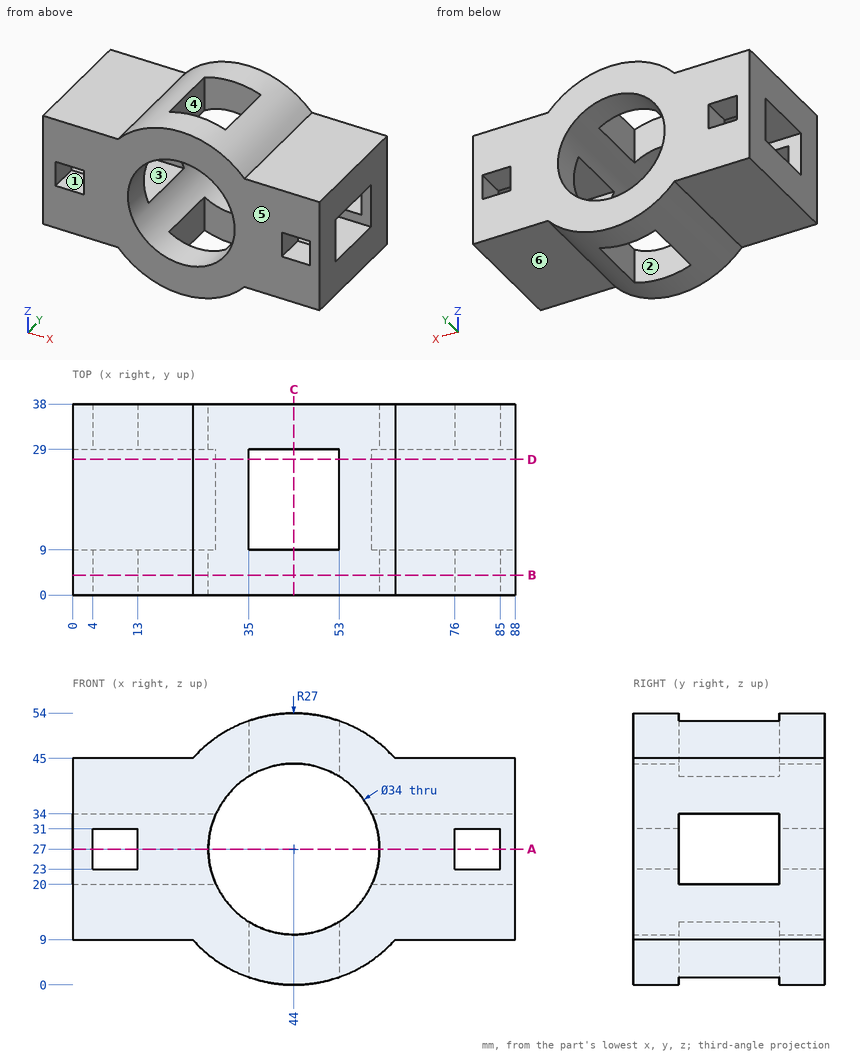
Job drawing, mm, ordinate dimensions from the low corner. One solid piece. A direction names the side the tool comes from. Give positions to 0.01 mm unless a question says otherwise; leave off trailing zeros. Loops run counter-clockwise (first coordinate to the right, second up) from the corner with the lowest first, then second, coordinate; pieces in that order, holes last.
Item 1: Flat gauge pins, fed straight in: pin 1 (4 mm diameter, centred on x = 40, z = 49, fed in from -Y); pin 2 (22 mm diameter, centred on x = 11, y = 19, fed in from +Z); pin 3 (4 mm diameter, centred on x = 42.5, y = 5, fed in from -Z); pin 4 (12 mm diameter, centred on x = 10, y = 22.5, fed in from -Z). Where does each tip first touch, or does it go through?
Answers follow:
pin 1: stops at y = 0
pin 2: stops at z = 45
pin 3: stops at z = 0
pin 4: stops at z = 9
Item 2: Slice it at D-D, the plane y = 27. List the corners of the cut face in (x, z).
Answers follow:
outline: (0, 9) - (23.88, 9) arc R27 ccw to (35, 1.54) - (35, 12.58) arc R17 cw to (28.51, 20) - (0, 20) - close; (0, 34) - (28.51, 34) arc R17 cw to (35, 41.42) - (35, 52.46) arc R27 ccw to (23.88, 45) - (0, 45) - close; (53, 1.54) arc R27 ccw to (64.12, 9) - (88, 9) - (88, 20) - (59.49, 20) arc R17 cw to (53, 12.58) - close; (53, 41.42) arc R17 cw to (59.49, 34) - (88, 34) - (88, 45) - (64.12, 45) arc R27 ccw to (53, 52.46) - close
Item 3: Slice it at B-B, the plane y = 4. List the corners of the cut face in (x, z).
Answers follow:
outline: (0, 9) - (23.88, 9) arc R27 ccw to (64.12, 9) - (88, 9) - (88, 45) - (64.12, 45) arc R27 ccw to (23.88, 45) - (0, 45) - close; hole (4, 23) - (13, 23) - (13, 31) - (4, 31) - close; hole circle Ø34 at (44, 27); hole (76, 23) - (85, 23) - (85, 31) - (76, 31) - close
Item 4: Slice it at A-A, the plane z = 27. Give the number of separate pieces and of enclosed holes in the cut face, and give its area (3 significant figures).
Answers follow:
separate pieces: 8
enclosed holes: 0
area: 648 mm2
Item 5: Which spindle directions (+Z, -Z, +X, -X, +Y, -Y) get a long thin tool onto all of the face, cutting with end or side? Do the marked faces 1, 2 and 3. Say none if no direction does.
Answers follow:
face 1: +Y, -Y
face 2: +Z, -Z
face 3: +X, -X
Item 6: Pull direction Y, two halves, no side cores. Call the marked faces 4, 5 and 6: released by +Y, released by -Y, zero draft, split by the parting line, or undercut.
Answers follow:
face 4: undercut
face 5: released by -Y
face 6: zero draft
Item 7: Slice it at C-C, the plane x = 44. List the corners of the cut face in (y, z).
Answers follow:
outline: (0, 0) - (9, 0) - (9, 10) - (0, 10) - close; (0, 44) - (9, 44) - (9, 54) - (0, 54) - close; (29, 0) - (38, 0) - (38, 10) - (29, 10) - close; (29, 44) - (38, 44) - (38, 54) - (29, 54) - close
Item 8: Drill centre lines: line 1 (X direction, y = 20, z = 11.5); line 2 (Y direction, x = 44.5, z = 3); line 3 (X direction, y = 35, z = 28.5). Where is each one in solid material? Low to high.
Answers follow:
line 1: x = 0 to 35, 53 to 88
line 2: y = 0 to 9, 29 to 38
line 3: x = 0 to 4, 13 to 27.07, 60.93 to 76, 85 to 88
